Check sheet for the drawn part. Datum: minimum x, y, z corner. Units: mm. Coordinates: 2 decimals unless noted, no trailing zeros. Write each loop counter-clockwise with the first axis right and the second up, starting at its lowest first coordinate (ties: lowest second). Pieces come first, ordered by that corner, then holes. Notation, with made-up numbers: M 57,-2.5 L 107,-2.5 A16 cw 107,8.5 Z; hole C 1,70.25 d2. An arc over 180 degrees is marked long. Answer as CSV lines item,"result". Start each with the question number.
Q1. Thickness scan on line 1 along Y through (x, z) = (2, 19); line 2 along Y through (x, z) = (12.5, 27) (1 decimal); line 3 along Z through (x, y) = (41, 26.5) (1 decimal). Record the ranges inside material, lowest first. Write a range as from..to.
Q2. Sectioned sample at A-A, the plane y = 19.05. Record the cut outline in (x, z), then the cut area to 3 significant figures.
Q3. Sectioned sample at B-B, the plane x = 81. Record the cut outline in (y, z).
Q4. Depth check by flat-ended pin: pin 1 Ø4 at (x, y) = (19.5, 32.5) entering from -Z (1 decimal); pin 2 Ø12 at (x, z) = (74.5, 23) entering from -Y; pin 3 Ø6 at (x, y) = (71, 31.5) entering from +Z; pin 4 Ø10 at (x, y) = (22.5, 27) entering from +Z. Enter the tip coordinate at first touch or a pass-through.
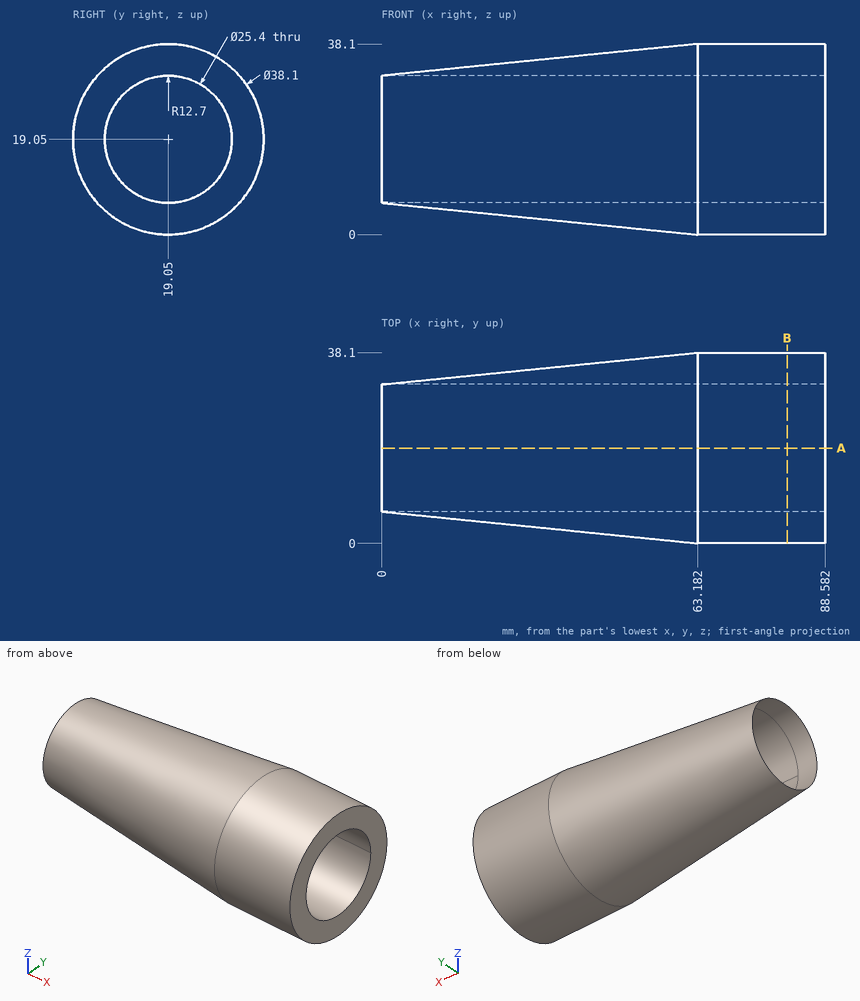
Output:
1,line 1,"y = 6.15..6.35, 31.75..31.95"
1,line 2,"y = 7.6..9.1, 29..30.5"
1,line 3,"z = 4..8.8, 29.3..34.1"
2,outline,"M 0,6.35 L 63.18,0 L 88.58,0 L 88.58,6.35 Z; M 0,31.75 L 88.58,31.75 L 88.58,38.1 L 63.18,38.1 Z"
2,area,"724 mm^2"
3,outline,"C 19.05,19.05 d38.1; hole C 19.05,19.05 d25.4"
4,pin 1,"stops at z = 9.9"
4,pin 2,"stops at y = 0"
4,pin 3,"stops at z = 35.59"
4,pin 4,"stops at z = 33.83"
